The listing builds one solid part. Answer for the finished solid, in the listing's coordinates (mm). Face numbers are marked on the shaded views. A direction names the side the tool comes from. Give positions to 0.01 mm unless a question says otherwise; leave off trailing zeros. Write each loop counter-clockwise with the first axis right and the second up, starting at its lowest first coordinate (ties: lowest second). Pieces come first, ordered by that corner, then holes. Notation, with made-up numbers: (0, 84) -> (10, 84) arc R19 ccw to (10, 115) -> close; hole circle Ø6 at (-34, 31). An arc over 180 degrees is marked (long way). Put each result on its own line as item: value. Start each with the question number.
1) A cutting plane is placed at C-C (y = 54). Write down the section's boundary in (x, z) (3 decimals).
2) A cutting plane is placed at A-A (z = -2). Write down the section's boundary in (x, y) (3 decimals).
3) A cutting plane is placed at B-B (x = 54). Write down the section's boundary in (y, z) (3 decimals).
4) Flat-ended cylindrical pins translate along their axes: pin 1 Ø2 at (y, z) = (-5, 11) entering from +X (3 decimals); pin 2 Ø1.5 at (x, z) = (-5.5, 30) entering from -Y; pin 3 Ø16.5 at (x, y) = (-18, 40) entering from +Z (3 decimals). Find the tip coordinate at first contact, or state that the pin passes through.
5) For the marked faces 5, 6, 7 and 8, determine the directions among +Z, -Z, +X, -X, +Y, -Y from which every point of the face is accessible in a straight line to the end or side of a thin tool.
6) Find the intervals of material crossed by line 1 along X through (y, z) = (21, 20) (3 decimals); line 2 along Z through (x, y) = (-34.5, -23.5) (3 decimals); line 3 along X through (y, z) = (-10.5, 7) (3 decimals), in increasing order. Write a range as from..to.
7) A cutting plane is placed at D-D (x = 70). Write down the section's boundary in (y, z) (3 decimals).
8) For a pull along X with two mould halves and no side action, classify the marked faces 1, 2, 3 and 4 as released by +X, released by -X, zero draft, split by the parting line, or undercut.
from build123d import *

# Parameters (mm, degrees)
F1_DEPTH = 63.5
F2_DEPTH = 25.4
F3_DEPTH = 7.9375
F5_R     = 5.08


with BuildPart() as f1:
    # F0 (on Front) → F1 (new body, symmetric)
    with BuildSketch(Plane.XZ):
        Polygon((-41.275, -9.525), (41.275, -9.525), (41.275, 9.525), (22.225, 9.525), (-41.275, 9.525), align=None)
    extrude(amount=F1_DEPTH, both=True)

    # F0 (on Front) → F2 (join, symmetric)
    with BuildSketch(Plane.XZ):
        with BuildLine():
            ThreePointArc((57.15, 61.9252), (52.3417131244, 61.5926269504), (47.625, 60.6012416505))
            Line((47.625, 60.6012416505), (47.625, 39.7002))
            ThreePointArc((47.625, 39.7002), (52.1298842145, 42.0605473566), (57.15, 42.8752))
            Line((57.15, 42.8752), (73.025, 42.8752))
            Line((73.025, 42.8752), (73.025, 61.9252))
            Line((73.025, 61.9252), (57.15, 61.9252))
        make_face()
        with BuildLine():
            Line((22.225, 9.525), (41.275, 9.525))
            Line((41.275, 9.525), (41.275, 27.0002))
            ThreePointArc((41.275, 27.0002), (42.9509683429, 34.0997158286), (47.625, 39.7002))
            Line((47.625, 39.7002), (47.625, 60.6012416505))
            ThreePointArc((47.625, 60.6012416505), (29.28948807, 48.0607674188), (22.225, 27.0002))
            Line((22.225, 27.0002), (22.225, 9.525))
        make_face()
    extrude(amount=F2_DEPTH, both=True)

    # F0 (on Front) → F3 (join, symmetric)
    with BuildSketch(Plane.XZ):
        with BuildLine():
            add(Edge.make_bspline(
                [(-41.275, 9.525), (-24.0416502966, 33.8548284783), (10.9341804068, 58.6884807018), (47.625, 60.6012416505)],
                knots=[0, 0, 0, 0, 102.5280081789, 102.5280081789, 102.5280081789, 102.5280081789], degree=3))
            Line((-41.275, 9.525), (22.225, 9.525))
            Line((22.225, 9.525), (22.225, 27.0002))
            ThreePointArc((22.225, 27.0002), (29.28948807, 48.0607674188), (47.625, 60.6012416505))
        make_face()
    extrude(amount=F3_DEPTH, both=True)

    # F0 (on Front) → F4 (revolve)
    with BuildSketch(Plane.XZ):
        Polygon((98.425, 66.675), (73.025, 66.675), (73.025, 61.9252), (73.025, 42.8752), (73.025, 38.1), (98.425, 38.1), align=None)
    revolve(axis=Axis((73.025, 0, 52.3875), (0, 0, 1)))

    # F5
    f5_edges = [f1.edges().sort_by_distance(p)[0] for p in [
        (-41.275, -63.5, 0),
        (-41.275, 63.5, 0),
        (41.275, 63.5, 0),
        (41.275, -63.5, 0),
    ]]
    fillet(f5_edges, radius=F5_R)


solid = f1.part
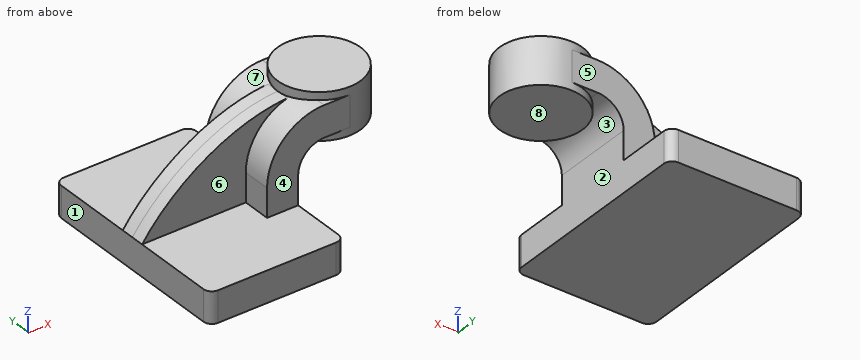
Reply:
1. outline: (-41.275, -9.525) -> (41.275, -9.525) -> (41.275, 9.525) -> (-41.275, 9.525) -> close
2. outline: (-41.275, -58.42) arc R5.08 ccw to (-36.195, -63.5) -> (36.195, -63.5) arc R5.08 ccw to (41.275, -58.42) -> (41.275, 58.42) arc R5.08 ccw to (36.195, 63.5) -> (-36.195, 63.5) arc R5.08 ccw to (-41.275, 58.42) -> close
3. outline: (-25.4, 42.56) -> (-16.829, 42.56) -> (-16.829, 38.1) -> (16.829, 38.1) -> (16.829, 42.56) -> (25.4, 42.56) -> (25.4, 61.783) -> (16.829, 61.783) -> (16.829, 66.675) -> (-16.829, 66.675) -> (-16.829, 61.783) -> (-25.4, 61.783) -> close
4. pin 1: stops at x = 41.275
4. pin 2: stops at y = -7.94
4. pin 3: stops at z = 9.525
5. face 5: +Z, +X, -X, +Y
5. face 6: +Z, -X, -Y
5. face 7: +Z, -X, +Y
5. face 8: -Z, +X, +Y, -Y
6. line 1: x = 22.225..41.275
6. line 2: z = -9.525..9.525
6. line 3: x = -41.275..41.275
7. outline: (-25.4, 42.875) -> (-25.219, 42.875) -> (-25.219, 38.1) -> (25.219, 38.1) -> (25.219, 42.875) -> (25.4, 42.875) -> (25.4, 61.925) -> (25.219, 61.925) -> (25.219, 66.675) -> (-25.219, 66.675) -> (-25.219, 61.925) -> (-25.4, 61.925) -> close
8. face 1: released by -X
8. face 2: released by +X
8. face 3: undercut
8. face 4: zero draft
